CAD build for the part. Positions are in the model's coordinates, mm. Face numbers are marked on the shaded views. A direction names the side the tool comes from. Coordinates: 2 decimals unless noted, no trailing zeros. Write each loop counter-clockwise with the first axis right and the second up, starting at its lowest first coordinate (ties: lowest second). Pieces come first, ordered by that corner, then holes. Notation, with made-up numbers: (72, 18.25) -> (90, 18.25) arc R25 cw to (90, 45.25) -> close; hole circle Ø4 at (50.25, 10.25). An arc over 180 degrees is marked (long way). Answer as CSV lines item,"result".
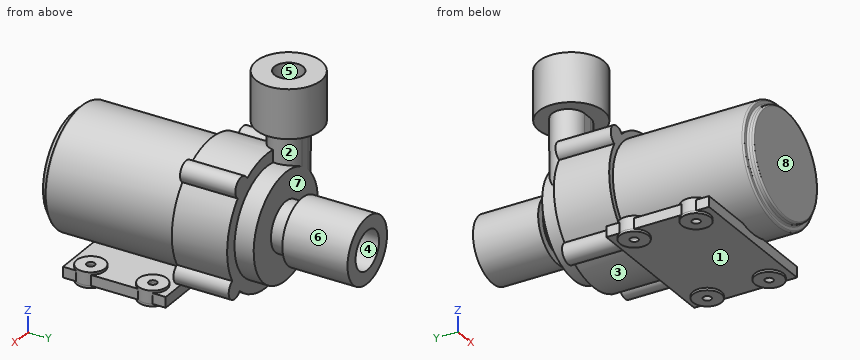
```python
from build123d import *

# Parameters (mm, degrees)
SKETCH1_R            = 18.415
BOSS_EXTRUDE1_DEPTH  = 42.672
SKETCH2_OUTSIDE_W    = 52.296
SKETCH2_OUTSIDE_H    = 52.296
SKETCH2_OUTSIDE_R    = 16.51
CUT_EXTRUDE2_DEPTH   = 1.9431
FILLET1_R            = 0.508
SKETCH3_W            = 45.212
SKETCH3_H            = 32.004
SKETCH3_R            = 1.27
BOSS_EXTRUDE2_DEPTH  = 2.54
SKETCH3_2_W          = 45.212
SKETCH3_2_H          = 32.004
SKETCH3_2_R          = 1.27
BOSS_EXTRUDE3_DEPTH  = 0.762
SKETCH5_R            = 4.445
SKETCH5_R_2          = 1.27
BOSS_EXTRUDE5_DEPTH  = 0.762
SKETCH5_4_R          = 4.445
SKETCH5_4_R_2        = 1.27
BOSS_EXTRUDE8_DEPTH  = 4.064
BOSS_EXTRUDE9_DEPTH  = 17.2339
SKETCH7_R            = 16.51
BOSS_EXTRUDE10_DEPTH = 5.969
SKETCH8_R            = 7.62
BOSS_EXTRUDE11_DEPTH = 5.08
SKETCH9_R            = 10.16
SKETCH9_R_2          = 6.0325
BOSS_EXTRUDE12_DEPTH = 20.32
BOSS_EXTRUDE13_START = -16.51
BOSS_EXTRUDE13_DEPTH = 16.51
BOSS_EXTRUDE14_DEPTH = 9.525
SKETCH11_R           = 10.16
SKETCH11_R_2         = 4.445
BOSS_EXTRUDE17_DEPTH = 15.24


with BuildPart() as part:
    # Sketch1 → Boss-Extrude1 (new body)
    with BuildSketch(Plane(origin=(0, 0, 0), x_dir=(1, 0, 0), z_dir=(0, 1, 0))):
        Circle(SKETCH1_R)
    extrude(amount=BOSS_EXTRUDE1_DEPTH)

    # Sketch2 outside → Cut-Extrude2 (cut)
    with BuildSketch(Plane.XZ):
        Rectangle(SKETCH2_OUTSIDE_W, SKETCH2_OUTSIDE_H)
        Circle(SKETCH2_OUTSIDE_R, mode=Mode.SUBTRACT)
    extrude(amount=-CUT_EXTRUDE2_DEPTH, mode=Mode.SUBTRACT)

    # Fillet1
    fillet1_edges = [part.edges().sort_by_distance(p)[0] for p in [
        (-16.51, 0, 0),
        (-16.51, 1.9431, 0),
        (-18.415, 1.9431, 0),
    ]]
    fillet(fillet1_edges, radius=FILLET1_R)



with BuildPart() as body_2:
    # Sketch3 → Boss-Extrude2 (new body)
    with BuildSketch(Plane(origin=(0, 0, -18.415), x_dir=(-1, 0, 0), z_dir=(0, 0, -1))):
        with Locations((0, 26.162)):
            Rectangle(SKETCH3_W, SKETCH3_H)
        with Locations((-18.796, 35.814)):
            Circle(SKETCH3_R, mode=Mode.SUBTRACT)
        with Locations((-18.796, 16.51)):
            Circle(SKETCH3_R, mode=Mode.SUBTRACT)
        with Locations((18.796, 16.51)):
            Circle(SKETCH3_R, mode=Mode.SUBTRACT)
        with Locations((18.796, 35.814)):
            Circle(SKETCH3_R, mode=Mode.SUBTRACT)
    extrude(amount=BOSS_EXTRUDE2_DEPTH)


with BuildPart() as part_1:
    add(part.part)

    add(body_2.part)  # Boss-Extrude3 merges body 2
    # Sketch3_2 → Boss-Extrude3 (add)
    with BuildSketch(Plane(origin=(0, 0, -18.415), x_dir=(-1, 0, 0), z_dir=(0, 0, -1))):
        with Locations((0, 26.162)):
            Rectangle(SKETCH3_2_W, SKETCH3_2_H)
        with Locations((-18.796, 35.814)):
            Circle(SKETCH3_2_R, mode=Mode.SUBTRACT)
        with Locations((-18.796, 16.51)):
            Circle(SKETCH3_2_R, mode=Mode.SUBTRACT)
        with Locations((18.796, 16.51)):
            Circle(SKETCH3_2_R, mode=Mode.SUBTRACT)
        with Locations((18.796, 35.814)):
            Circle(SKETCH3_2_R, mode=Mode.SUBTRACT)
    extrude(amount=-BOSS_EXTRUDE3_DEPTH)

    # Sketch5 → Boss-Extrude5 (add)
    with BuildSketch(Plane(origin=(0, 0, -20.955), x_dir=(-1, 0, 0), z_dir=(0, 0, -1))):
        with Locations((-18.796, 35.814)):
            Circle(SKETCH5_R)
        with Locations((-18.796, 35.814)):
            Circle(SKETCH5_R_2, mode=Mode.SUBTRACT)
        with Locations((-18.796, 16.51)):
            Circle(SKETCH5_R)
        with Locations((-18.796, 16.51)):
            Circle(SKETCH5_R_2, mode=Mode.SUBTRACT)
        with Locations((18.796, 16.51)):
            Circle(SKETCH5_R)
        with Locations((18.796, 16.51)):
            Circle(SKETCH5_R_2, mode=Mode.SUBTRACT)
        with Locations((18.796, 35.814)):
            Circle(SKETCH5_R)
        with Locations((18.796, 35.814)):
            Circle(SKETCH5_R_2, mode=Mode.SUBTRACT)
    extrude(amount=BOSS_EXTRUDE5_DEPTH)

    # Sketch5_4 → Boss-Extrude8 (add)
    with BuildSketch(Plane(origin=(0, 0, -20.955), x_dir=(-1, 0, 0), z_dir=(0, 0, -1))):
        with Locations((-18.796, 35.814)):
            Circle(SKETCH5_4_R)
        with Locations((-18.796, 35.814)):
            Circle(SKETCH5_4_R_2, mode=Mode.SUBTRACT)
        with Locations((-18.796, 16.51)):
            Circle(SKETCH5_4_R)
        with Locations((-18.796, 16.51)):
            Circle(SKETCH5_4_R_2, mode=Mode.SUBTRACT)
        with Locations((18.796, 16.51)):
            Circle(SKETCH5_4_R)
        with Locations((18.796, 16.51)):
            Circle(SKETCH5_4_R_2, mode=Mode.SUBTRACT)
        with Locations((18.796, 35.814)):
            Circle(SKETCH5_4_R)
        with Locations((18.796, 35.814)):
            Circle(SKETCH5_4_R_2, mode=Mode.SUBTRACT)
    extrude(amount=-BOSS_EXTRUDE8_DEPTH)

    # Sketch6 → Boss-Extrude9 (add)
    with BuildSketch(Plane(origin=(0, 42.672, 0), x_dir=(1, 0, 0), z_dir=(0, 1, 0))):
        with BuildLine():
            ThreePointArc((-14.885846945, 13.831628998), (-20.183913314, 2.347774127), (-17.663218531, -10.045551809))
            ThreePointArc((-17.663218531, -10.045551809), (-18.820039984, -14.897989932), (-13.831628998, -14.885846945))
            ThreePointArc((-13.831628998, -14.885846945), (-2.347774127, -20.183913314), (10.045551809, -17.663218531))
            ThreePointArc((10.045551809, -17.663218531), (14.897989932, -18.820039984), (14.885846945, -13.831628998))
            ThreePointArc((14.885846945, -13.831628998), (20.183913314, -2.347774127), (17.663218531, 10.045551809))
            ThreePointArc((17.663218531, 10.045551809), (18.820039984, 14.897989932), (13.831628998, 14.885846945))
            ThreePointArc((13.831628998, 14.885846945), (2.347774127, 20.183913314), (-10.045551809, 17.663218531))
            ThreePointArc((-10.045551809, 17.663218531), (-14.897989932, 18.820039984), (-14.885846945, 13.831628998))
        make_face()
    extrude(amount=BOSS_EXTRUDE9_DEPTH)

    # Sketch7 → Boss-Extrude10 (add)
    with BuildSketch(Plane(origin=(0, 59.9059, 0), x_dir=(1, 0, 0), z_dir=(0, 1, 0))):
        Circle(SKETCH7_R)
    extrude(amount=BOSS_EXTRUDE10_DEPTH)

    # Sketch8 → Boss-Extrude11 (add)
    with BuildSketch(Plane(origin=(0, 65.8749, 0), x_dir=(1, 0, 0), z_dir=(0, 1, 0))):
        Circle(SKETCH8_R)
    extrude(amount=BOSS_EXTRUDE11_DEPTH)

    # Sketch9 → Boss-Extrude12 (add)
    with BuildSketch(Plane(origin=(0, 70.9549, 0), x_dir=(1, 0, 0), z_dir=(0, 1, 0))):
        Circle(SKETCH9_R)
        Circle(SKETCH9_R_2, mode=Mode.SUBTRACT)
    extrude(amount=BOSS_EXTRUDE12_DEPTH)

    # Sketch10 → Boss-Extrude13 (add)
    with BuildSketch(Plane.XY.offset(16.51).offset(BOSS_EXTRUDE13_START)):
        with BuildLine():
            Line((-8.382, 65.8749), (-11.43, 65.8749))
            ThreePointArc((-11.43, 65.8749), (-16.51, 60.7949), (-11.43, 55.7149))
            Line((-11.43, 55.7149), (-8.382, 55.7149))
            ThreePointArc((-8.382, 55.7149), (-3.302, 60.7949), (-8.382, 65.8749))
        make_face()
    extrude(amount=BOSS_EXTRUDE13_DEPTH)

    # Sketch10_2 → Boss-Extrude14 (add)
    with BuildSketch(Plane.XY.offset(16.51)):
        with BuildLine():
            Line((-11.43, 65.8749), (-8.382, 65.8749))
            ThreePointArc((-8.382, 65.8749), (-3.302, 60.7949), (-8.382, 55.7149))
            Line((-8.382, 55.7149), (-11.43, 55.7149))
            ThreePointArc((-11.43, 55.7149), (-16.51, 60.7949), (-11.43, 65.8749))
        make_face()
    extrude(amount=BOSS_EXTRUDE14_DEPTH)

    # Sketch11 → Boss-Extrude17 (add)
    with BuildSketch(Plane.XY.offset(26.035)):
        with Locations((-9.906, 60.7949)):
            Circle(SKETCH11_R)
        with Locations((-9.906, 60.7949)):
            Circle(SKETCH11_R_2, mode=Mode.SUBTRACT)
    extrude(amount=BOSS_EXTRUDE17_DEPTH)


solid = part_1.part
```
Item 1: 3-axis set-ups, long thin cutter, end or side, ignore diameter. For the marked faces 1, 2, 3, 4 and 5: which of +Z, -Z, +X, -X, +Y, -Y reach the whole face in a straight line?
Answer below:
face 1,"-Z"
face 2,"none"
face 3,"-Z, +Y"
face 4,"+Y"
face 5,"+Z"
Item 2: Flat gauge pins, fed straight in: pin 1 (1.7 mm diameter, centred on y = 40.5, z = -19.5, fed in from -X); pin 2 (3.5 mm diameter, centred on x = -8, z = -19.5, fed in from +Y); pin 3 (2.5 mm diameter, centred on x = -11.5, y = 60, fed in from +Z) (3 decimals). Where does each tip first touch, or does it go through?
Answer below:
pin 1,"stops at x = -22.61"
pin 2,"stops at y = 59.91"
pin 3,"stops at z = 26.035"
Item 3: Saw through at B-B on y = 27.5. Give the cut face in (x, z) (1 decimal), and give its area (3 significant figures).
Answer below:
outline,"(-22.6, -21) -> (22.6, -21) -> (22.6, -17.7) -> (5.2, -17.7) arc R18.4 ccw (long way) to (-5.2, -17.7) -> (-22.6, -17.7) -> close"
area,"1,210 mm2"
Item 4: Saw through at D-D on y = 57.5. Give the cut face in (x, z) (3 decimals).
Answer below:
outline,"(-19.517, 26.035) -> (-15.297, 26.035) -> (-15.297, 15.929) arc R3.175 ccw to (-17.663, 10.046) arc R20.32 ccw to (-14.886, -13.832) arc R3.175 ccw (long way) to (-10.046, -17.663) arc R20.32 ccw to (13.832, -14.886) arc R3.175 ccw (long way) to (17.663, -10.046) arc R20.32 ccw to (14.886, 13.832) arc R3.175 ccw (long way) to (10.046, 17.663) arc R20.32 ccw to (-4.515, 19.812) -> (-4.515, 26.035) -> (-0.295, 26.035) -> (-0.295, 41.275) -> (-6.922, 41.275) -> (-6.922, 26.035) -> (-12.89, 26.035) -> (-12.89, 41.275) -> (-19.517, 41.275) -> close"
Item 5: Wall check: line 1 (Y direction, x = -1.5, z = -18); line 2 (Y direction, x = 16, z = 0); line 3 (Y direction, x = 18, z = -19). Give the ranges that are in metal, low to high. Write a range as from..to.
Answer below:
line 1,"y = 1.97..59.91"
line 2,"y = 0..65.87"
line 3,"y = 10.16..15.52, 17.5..34.82, 36.8..42.16"
Item 6: Saw through at C-C on z = 37. Give the cut face in (x, y) (3 decimals), and give its area (3 significant figures).
Answer below:
outline,"circle Ø20.32 at (-9.906, 60.795); hole circle Ø8.89 at (-9.906, 60.795)"
area,"262 mm2"
Item 7: Saw through at A-A on y = 16.51. Give the cut face in (x, z) (1 decimal).
Answer below:
outline,"(-23.2, -21.7) -> (-20.1, -21.7) -> (-20.1, -16.9) -> (-23.2, -16.9) -> close; (-17.5, -21.7) -> (-14.4, -21.7) -> (-14.4, -21) -> (14.4, -21) -> (14.4, -21.7) -> (17.5, -21.7) -> (17.5, -16.9) -> (14.4, -16.9) -> (14.4, -17.7) -> (5.2, -17.7) arc R18.4 ccw (long way) to (-5.2, -17.7) -> (-14.4, -17.7) -> (-14.4, -16.9) -> (-17.5, -16.9) -> close; (20.1, -21.7) -> (23.2, -21.7) -> (23.2, -16.9) -> (20.1, -16.9) -> close"
Item 8: Two-plate mould, pull along Y, no slides. Class the marked faces 6, 7 and 8: pulls with the +Y half, pulls with the -Y half, needs draft (parallel to the pull), parting line crosses it, or undercut.
Answer below:
face 6,"needs draft"
face 7,"undercut"
face 8,"pulls with the -Y half"
